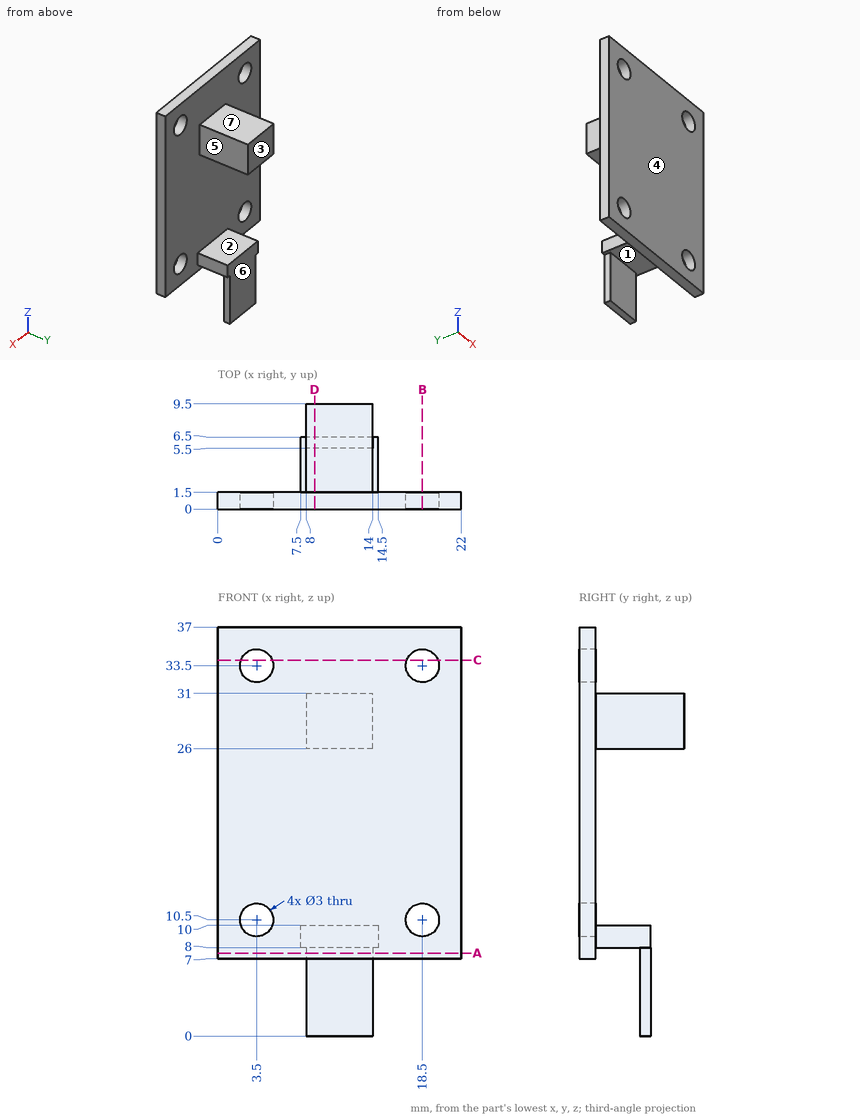
Job drawing, mm, ordinate dimensions from the low corner. One solid piece. A direction names the side the tool comes from. Give positions to 0.01 mm unless a question says otherwise; leave off trailing zeros. Order: outer loops, then holes, each group sorted by start corner. A loop starts at its lowest first (then second) coordinate and runs counter-clockwise, first axis right, second up. Notation, with made-up numbers: M -33.5,11.5 L -10.5,11.5 A31 cw -10.5,49.5 Z; hole C 32.5,15 d6. An arc over 180 degrees is marked long. Put each result on its own line as item: value. Start each with the question number.
(1) Band-saw the part on B-B on x = 18.5. Give the cut face in (y, z), then the cut area to 3 significant figures.
(2) Pin check, flat tips, straight feed: pin 1 Ø5.5 at (y, z) = (4.5, 28) entering from -X; pin 2 Ø5.5 at (x, z) = (9.5, 6) entering from +Y; pin 3 Ø6.5 at (x, z) = (12, 3.5) entering from -Y; pin 4 Ø2.5 at (x, z) = (18.5, 33.5) entering from +Y. Stop position of each tip, or through.
(3) Band-saw the part on C-C on z = 34. Give the cut face in (x, y), then the cut area to 3 significant figures.
(4) Tool access for the marked faces 5, 6 and 7: list every direction of +Z, -Z, +X, -X, +Y, -Y with a clear straight run to the whole face (end or side of a thin tool).
(5) Band-saw the part on A-A on z = 7.5. Give the cut face in (x, y).
(6) Pull direction Y, two halves, no side cores. Call the marked faces 1, 2, 3 and 4: released by +Y, released by -Y, zero draft, split by the parting line, or undercut.
(7) Band-saw the part on D-D on x = 8.75. Give the cut face in (y, z).
(8) Drill centre lines: L1, parallel to Z at x = 18.5, y = 1.15; L2, parallel to Z at x = 9, y = 4.75; L3, parallel to X at y = 0.75, z = 32.5. Where is each one in solid material? Low to high. Write a range as [from, to].
Results below:
1. outline: M 0,7 L 1.5,7 L 1.5,9 L 0,9 Z; M 0,12 L 1.5,12 L 1.5,32 L 0,32 Z; M 0,35 L 1.5,35 L 1.5,37 L 0,37 Z
1. area: 36.0 mm2
2. pin 1: stops at x = 8
2. pin 2: stops at y = 6.5
2. pin 3: stops at y = 5.5
2. pin 4: passes through
3. outline: M 0,0 L 2.09,0 L 2.09,1.5 L 0,1.5 Z; M 4.91,0 L 17.09,0 L 17.09,1.5 L 4.91,1.5 Z; M 19.91,0 L 22,0 L 22,1.5 L 19.91,1.5 Z
3. area: 24.5 mm2
4. face 5: +Z, +X, +Y
4. face 6: -Z, +X, -X, +Y
4. face 7: +Z, +X, -X, +Y
5. outline: M 0,0 L 22,0 L 22,1.5 L 0,1.5 Z; M 8,5.5 L 14,5.5 L 14,6.5 L 8,6.5 Z
6. face 1: undercut
6. face 2: zero draft
6. face 3: released by +Y
6. face 4: released by -Y
7. outline: M 0,7 L 1.5,7 L 1.5,8 L 5.5,8 L 5.5,0 L 6.5,0 L 6.5,10 L 1.5,10 L 1.5,26 L 9.5,26 L 9.5,31 L 1.5,31 L 1.5,37 L 0,37 Z
8. L1: z = [7, 9], [12, 32], [35, 37]
8. L2: z = [8, 10], [26, 31]
8. L3: x = [0, 2.38], [4.62, 17.38], [19.62, 22]
